Can you work these out from the model? Positions are in its coordinate system, mm. Round coordinates to 2 decimals unless told otherwise and drop trailing zeros. Answer as a JSON object with one key per item and string values. Group by question number.
```python
from build123d import *

# Parameters (mm, degrees)
EXTRUDE_1_DEPTH        = 280
PATTERN_LINEAR_1_COUNT = 14
PATTERN_LINEAR_1_PITCH = 20


with BuildPart() as part:
    # 草图2 → 凸台-拉伸1 (new body)
    with BuildSketch(Plane.XY):
        with BuildLine():
            Line((4.1775, 6.5), (-4.1775, 6.5))
            Line((-4.1775, 6.5), (-4.5, 6.1775))
            Line((-4.5, 6.1775), (-4.5, 5.10375))
            ThreePointArc((-4.5, 5.10375), (-4.185793433, 4.9227306), (-3.986173862, 4.62))
            Line((-3.986173862, 4.62), (-3.626173862, 4.62))
            ThreePointArc((-3.626173862, 4.62), (-3.562534251, 4.59363961), (-3.536173862, 4.53))
            Line((-3.536173862, 4.53), (-3.536173862, 4.17))
            ThreePointArc((-3.536173862, 4.17), (-3.562534251, 4.10636039), (-3.626173862, 4.08))
            Line((-3.626173862, 4.08), (-3.986173862, 4.08))
            ThreePointArc((-3.986173862, 4.08), (-4.185793433, 3.7772694), (-4.5, 3.59625))
            Line((-4.5, 3.59625), (-4.5, 0.3225))
            Line((-4.5, 0.3225), (-4.1775, 0))
            Line((-4.1775, 0), (4.1775, 0))
            Line((4.1775, 0), (4.5, 0.3225))
            Line((4.5, 0.3225), (4.5, 3.59625))
            ThreePointArc((4.5, 3.59625), (4.185793433, 3.7772694), (3.986173862, 4.08))
            Line((3.986173862, 4.08), (3.626173862, 4.08))
            ThreePointArc((3.626173862, 4.08), (3.562534251, 4.10636039), (3.536173862, 4.17))
            Line((3.536173862, 4.17), (3.536173862, 4.53))
            ThreePointArc((3.536173862, 4.53), (3.562534251, 4.59363961), (3.626173862, 4.62))
            Line((3.626173862, 4.62), (3.986173862, 4.62))
            ThreePointArc((3.986173862, 4.62), (4.185793433, 4.9227306), (4.5, 5.10375))
            Line((4.5, 5.10375), (4.5, 6.1775))
            Line((4.5, 6.1775), (4.1775, 6.5))
        make_face()
    extrude(amount=-EXTRUDE_1_DEPTH)

    # 草图3 → 切除-旋转1 (revolve, cut)
    with BuildSketch(Plane(origin=(0, 0, 0), x_dir=(0, 0, -1), z_dir=(1, 0, 0))):
        Polygon((7, 6.5), (7, 3), (8.25, 3), (8.25, 0), (10, 0), (10, 6.5), align=None)
    cut_revolve_1 = revolve(axis=Axis((0, 6.5, -10), (0, -1, 0)), mode=Mode.SUBTRACT)

    # 阵列(线性)1: 切除-旋转1 ×14
    with Locations(*[(0, 0, -i * PATTERN_LINEAR_1_PITCH) for i in range(1, PATTERN_LINEAR_1_COUNT)]):
        add(cut_revolve_1, mode=Mode.SUBTRACT)


solid = part.part
```
1) For pin 1 (4.5 mm diameter, centred on x = 0, z = -250, fed in from +Y); pin 2 (3 mm diameter, centred on x = 0, z = -230, fed in from -Y); pin 3 (3 mm diameter, centred on x = 3, z = -58.5, fed in from -Y), each with a flat end and sliding along its axis, tell me the tip position at first contact or that it passes through.
2) I need wall thicknesses on line 1 along X through (y, z) = (4.65, -150); line 2 along X through (y, z) = (1.8, -150); line 3 along Y through (x, z) = (-0.75, -112.5). Which ranges of each line are inside material? Lowest first, please.
3) If we section it at B-B on x = 0: Count the separate pieces of the cut face and the enclosed holes in it, plus the area to 3 significant figures.
Findings:
{
 "1": {"pin 1": "stops at y = 3", "pin 2": "passes through", "pin 3": "stops at y = 0"},
 "2": {"line 1": "x = -4 to -3, 3 to 4", "line 2": "x = -4.5 to -1.75, 1.75 to 4.5", "line 3": "y = 0 to 3"},
 "3": {"separate pieces": "15", "enclosed holes": "0", "area": "1,380 mm^2"}
}
